Input: part model. Units: mm. Frame: model coordinates. A direction names the side the tool comes from. Round coordinates to 2 decimals unless told otherwise and drop trailing zeros. Order: outer loops, then holes, each group sorted by start corner. A loop starts at its lowest first (then second) coordinate and runs counter-clockwise, first axis right, second up.
Item 1: Reachability of faces 1 (the flat face through (-28.205, -6, 41)), 2 (the flat face through (-53.605, -6, 41)), 3 (the flat face through (-41, -31.75, 9)), 4 (the cylindrical face through (-28.06, -21.27, 9.36)), 5 (the flat face through (-41, -22, 12.584)) from +Z, -Z, +X, -X, +Y, -Y: full face, straight path, thin tool, end or side. Return the list, or none.
Item 2: Cut plane C-C on z = 62.5. Output: boundary loops of the cut face in (x, y), then the cut area to 3 significant figures.
Item 3: Cut plane B-B on x = -43. Output: boundary loops of the cut face in (y, z), then the cut area to 3 significant figures.
Item 4: First-contact query: pin 1 (8.5 mm diameter, centred on x = -25.03, y = -22.22, fed in from -Z); pin 2 (9.5 mm diameter, centred on x = -31, y = -20.5, fed in from +Z); pin 3 (4 mm diameter, centred on y = -7, z = 17.5, fed in from -X); pin 4 (3 mm diameter, centred on x = -33, y = -11, fed in from +Z). Flat tips, straight axial feed; report the tip coordinate or a pass-through.
Item 5: Cut plane D-D on x = -49. Output: boundary loops of the cut face in (y, z).
Item 6: Mould query, pull axis Z, two halves, no side actions, for faces 6 (the flat face through (-41, -12.7, 30)), 7 (the cylindrical face through (-16.95, -30.22, 9.45)), 8 (the flat face through (-41, -16, 6.234)). Classes: released by +Z, released by -Z, zero draft, split by the parting line, or undercut.
Item 7: Line query: L1, parallel to Z at x = -43.5, y = -24; L2, parallel to X at y = -21.5, z = 11.5; L3, parallel to Y at x = -21.5, z = 12.5. Output: solid intervals per line, ascending.
Item 8: Cut plane A-A on y = -23. Output: boundary loops of the cut face in (x, z).
```python
from build123d import *

# Parameters (mm, degrees)
F0_W     = 50.8
F0_H     = 52.8410717415
F0_H_2   = 10.6589282585
F1_DEPTH = 12.7
F2_W     = 50.8
F2_H     = 6.35
F3_DEPTH = 19.05
F5_DEPTH = 25.4
F7_DEPTH = 25.4
F9_D     = 12.7
F10_R    = 5.08
F12_D    = 6.35


with BuildPart() as f1:
    # F0 (on Front) → F1 (new body)
    with BuildSketch(Plane.XZ):
        with Locations((-40.9050544952, 43.3130595229)):
            Rectangle(F0_W, F0_H)
        with Locations((-40.9050544952, 11.5630595229)):
            Rectangle(F0_W, F0_H_2)
    extrude(amount=F1_DEPTH)

    # F2 (on face) → F3 (join)
    with BuildSketch(Plane.XZ.offset(12.7)):
        with Locations((-40.9050544952, 9.4085953936)):
            Rectangle(F2_W, F2_H)
    extrude(amount=F3_DEPTH)

    # F4 (on face) → F5 (cut)
    with BuildSketch(Plane.XZ.offset(12.7)):
        with BuildLine():
            Line((-53.6050544952, 25.2835953936), (-53.6050544952, 57.0335953936))
            ThreePointArc((-53.6050544952, 57.0335953936), (-49.8853106163, 66.0138515147), (-40.9050544952, 69.7335953936))
            Line((-40.9050544952, 69.7335953936), (-66.3050544952, 69.7335953936))
            Line((-66.3050544952, 69.7335953936), (-66.3050544952, 12.5835953936))
            ThreePointArc((-66.3050544952, 12.5835953936), (-57.3247983741, 16.3033392725), (-53.6050544952, 25.2835953936))
        make_face()
        with BuildLine():
            ThreePointArc((-40.9050544952, 69.7335953936), (-31.9247983741, 66.0138515147), (-28.2050544952, 57.0335953936))
            Line((-28.2050544952, 57.0335953936), (-28.2050544952, 25.2835953936))
            ThreePointArc((-28.2050544952, 25.2835953936), (-24.4853106163, 16.3033392725), (-15.5050544952, 12.5835953936))
            Line((-15.5050544952, 12.5835953936), (-15.5050544952, 69.7335953936))
            Line((-15.5050544952, 69.7335953936), (-40.9050544952, 69.7335953936))
        make_face()
    extrude(amount=-F5_DEPTH, mode=Mode.SUBTRACT)

    # F6 (on face) → F7 (join)
    with BuildSketch(Plane.XZ.offset(12.7)):
        with BuildLine():
            ThreePointArc((-53.6050544952, 57.0335953936), (-40.9050544952, 44.3335953936), (-28.2050544952, 57.0335953936))
            ThreePointArc((-28.2050544952, 57.0335953936), (-40.9050544952, 69.7335953936), (-53.6050544952, 57.0335953936))
        make_face()
    extrude(amount=F7_DEPTH)

    # F9 (through all)
    with Locations(Plane.XZ.offset(38.1)):
        with Locations((-40.9050544952, 57.0335953936)):
            Hole(F9_D / 2)

    # F10
    f10_edges = [f1.edges().sort_by_distance(p)[0] for p in [
        (-66.305054, -31.75, 9.408595),
        (-15.505054, -31.75, 9.408595),
    ]]
    fillet(f10_edges, radius=F10_R)

    # F12 (through all)
    with Locations(Plane.XY.offset(12.5835953936)):
        with Locations((-56.7800544952, -22.225), (-25.0300544952, -22.225)):
            Hole(F12_D / 2)


solid = f1.part
```
From the geometry:
1. face 1: +Z, +X, +Y, -Y
1. face 2: +Z, -X, +Y, -Y
1. face 3: -Z, +X, -X, -Y
1. face 4: +Z, -Z
1. face 5: +X, -X, -Y
2. outline: (-52.37, -38.1) - (-44.14, -38.1) - (-44.14, 0) - (-52.37, 0) - close; (-37.67, -38.1) - (-29.44, -38.1) - (-29.44, 0) - (-37.67, 0) - close
2. area: 627 mm2
3. outline: (-38.1, 44.51) - (-12.7, 44.51) - (-12.7, 12.58) - (-31.75, 12.58) - (-31.75, 6.23) - (0, 6.23) - (0, 51.04) - (-38.1, 51.04) - close; (-38.1, 63.03) - (0, 63.03) - (0, 69.56) - (-38.1, 69.56) - close
3. area: 1,100 mm2
4. pin 1: stops at z = 6.23
4. pin 2: stops at z = 68.64
4. pin 3: stops at x = -58.21
4. pin 4: stops at z = 68
5. outline: (-38.1, 47.25) - (-12.7, 47.25) - (-12.7, 12.58) - (-31.75, 12.58) - (-31.75, 6.23) - (0, 6.23) - (0, 66.82) - (-38.1, 66.82) - close
6. face 6: undercut
6. face 7: zero draft
6. face 8: released by -Z
7. L1: z = 6.23 to 12.58, 44.6 to 51.24, 62.83 to 69.47
7. L2: x = -66.31 to -59.87, -53.69 to -28.12, -21.94 to -15.51
7. L3: y = -31.75 to 0
8. outline: (-66.31, 6.23) - (-59.86, 6.23) - (-59.86, 12.58) - (-66.31, 12.58) - close; (-53.7, 6.23) - (-28.11, 6.23) - (-28.11, 12.58) - (-53.7, 12.58) - close; circle Ø25.4 at (-40.91, 57.03); (-21.95, 6.23) - (-15.51, 6.23) - (-15.51, 12.58) - (-21.95, 12.58) - close; hole circle Ø12.7 at (-40.91, 57.03)
